The model under review builds one solid part; all positions refer to its coordinate system, in mm. A direction names the side the tool comes from. Coordinates: 2 decimals unless noted, no trailing zeros. Write each loop counter-clockwise with the first axis right and the second up, starting at its lowest first coordinate (ties: lowest second). Pieces come first, ordered by that corner, then holes. Notation, with made-up numbers: (88, 67.25) - (103, 67.25) arc R29 ccw to (103, 103.25) - close; hole circle Ø11 at (1.25, 68). An arc over 180 degrees is marked (long way). Put each result on its own line as item: value.
from build123d import *

# Parameters (mm, degrees)
SKETCH1_R           = 3
BOSS_EXTRUDE1_DEPTH = 9.5
SKETCH2_R           = 2.25
CUT_EXTRUDE1_DEPTH  = 3.5
SKETCH3_R           = 1.25
CUT_EXTRUDE2_DEPTH  = 6
FILLET1_R           = 0.15
FILLET2_R           = 0.3


with BuildPart() as part:
    # Sketch1 → Boss-Extrude1 (new body)
    with BuildSketch(Plane.XY):
        Circle(SKETCH1_R)
    extrude(amount=BOSS_EXTRUDE1_DEPTH)

    # Sketch2 → Cut-Extrude1 (cut)
    with BuildSketch(Plane.XY.offset(9.5)):
        Circle(SKETCH2_R)
    extrude(amount=-CUT_EXTRUDE1_DEPTH, mode=Mode.SUBTRACT)

    # Sketch3 → Cut-Extrude2 (cut)
    with BuildSketch(Plane.XY.offset(6)):
        Circle(SKETCH3_R)
    extrude(amount=-CUT_EXTRUDE2_DEPTH, mode=Mode.SUBTRACT)

    # Fillet1
    fillet1_edges = [part.edges().sort_by_distance(p)[0] for p in [
        (-3, 0, 9.5),
        (-2.25, 0, 9.5),
    ]]
    fillet(fillet1_edges, radius=FILLET1_R)

    # Fillet2
    fillet2_edges = [part.edges().sort_by_distance(p)[0] for p in [
        (-3, 0, 0),
    ]]
    fillet(fillet2_edges, radius=FILLET2_R)


solid = part.part
1. To check wall thickness, follow probe 1 along Y at (x, z) = (0, 1.35); probe 2 along Y at (x, z) = (0, 6.9); probe 3 along X at (y, z) = (1, 4.75). State the ranges of each line that lie inside material, in increasing order.
Determined:
probe 1: y = -3 to -1.25, 1.25 to 3
probe 2: y = -3 to -2.25, 2.25 to 3
probe 3: x = -2.83 to -0.75, 0.75 to 2.83
2. Consider section A-A on y = 0. State the section outline as (x, z) points.
Determined:
outline: (-3, 0.3) arc R0.3 ccw to (-2.7, 0) - (-1.25, 0) - (-1.25, 6) - (-2.25, 6) - (-2.25, 9.35) arc R0.15 ccw to (-2.4, 9.5) - (-2.85, 9.5) arc R0.15 ccw to (-3, 9.35) - close; (1.25, 0) - (2.7, 0) arc R0.3 ccw to (3, 0.3) - (3, 9.35) arc R0.15 ccw to (2.85, 9.5) - (2.4, 9.5) arc R0.15 ccw to (2.25, 9.35) - (2.25, 6) - (1.25, 6) - close
3. For pin 1 Ø1 at (y, z) = (-2.5, 3) entering from -X; pin 2 Ø2 at (y, z) = (2, 2.5) entering from -X; pin 3 Ø1.3 at (x, y) = (0, 0.5) entering from +Z; pin 4 Ø3 at (x, y) = (0, 0) entering from +Z, all flat-tipped, find the tip position at first contact; note any pin that passes through.
Determined:
pin 1: stops at x = -2.24
pin 2: stops at x = -2.83
pin 3: passes through
pin 4: stops at z = 6
4. The part is to be moulded in two halves that separate along X. For faces 3 (the flat face through (1, -1, 0)), 4 (the cylindrical face through (-3, 0, 5)), 5 (the cylindrical face through (-0.29, 2.23, 7.7)), say which applies: +X half, -X half, draft (parallel to the pull), parting line (faces both ways), or undercut.
Determined:
face 3: draft
face 4: parting line
face 5: undercut
5. Consider section D-D on z = 3. State the section outline as (x, y) points, plus the area to 3 significant figures.
Determined:
outline: circle Ø6 at (0, 0); hole circle Ø2.5 at (0, 0)
area: 23.4 mm^2
6. Consider section C-C on z = 6.5. State the section outline as (x, y) points, plus the area to 3 significant figures.
Determined:
outline: circle Ø6 at (0, 0); hole circle Ø4.5 at (0, 0)
area: 12.4 mm^2
7. Machinability: for faces 1 (the cylindrical face through (-0.27, -1.22, 3.04)), 2 (the flat face through (1, -1, 6)), which of the approach directions +Z, -Z, +X, -X, +Y, -Y give a long, thin tool a straight path to every point of the face, cutting with its end or side? Answer none if there is none.
Determined:
face 1: +Z, -Z
face 2: +Z
